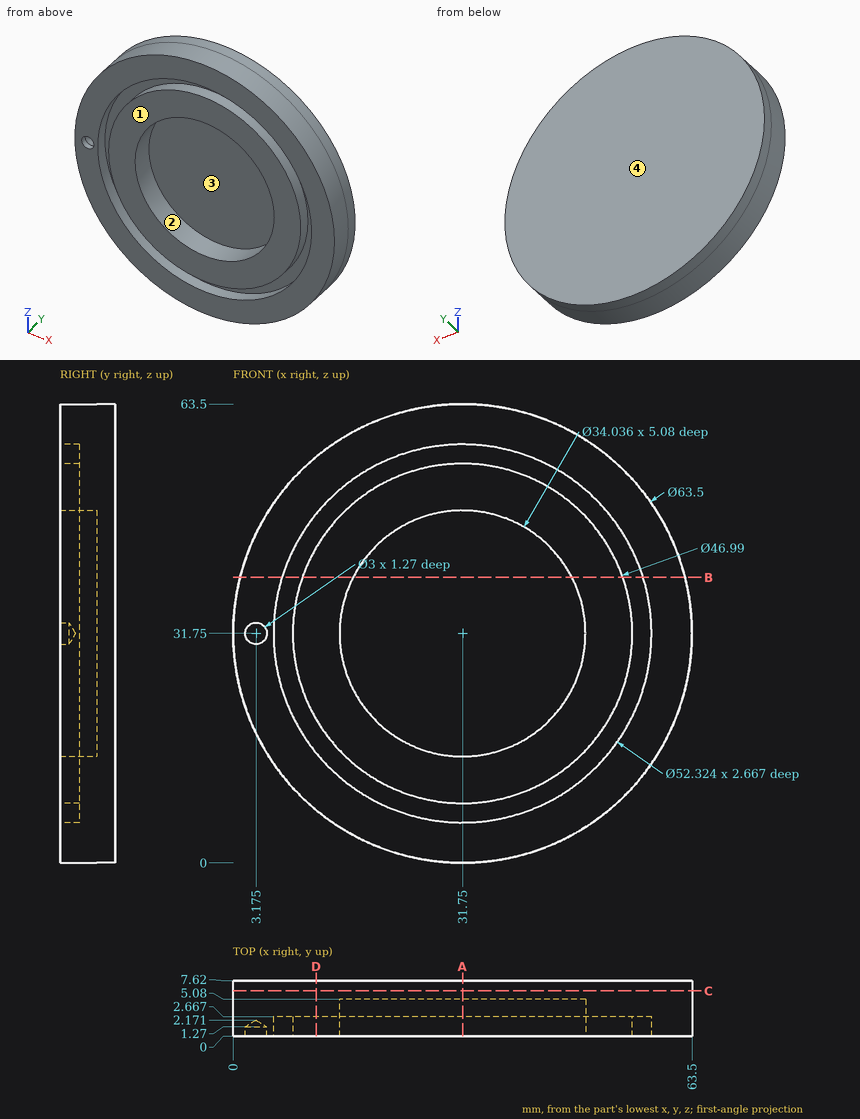
Geometry: see drawing. Coordinates: mm, zero at the bounding-box minimum. A direction names the side the tool comes from. Coordinates: 2 decimals unless noted, no trailing zeros. Order: outer loops, then holes, each group sorted by start corner. A loop starts at its lowest first (then second) coordinate and runs counter-clockwise, first axis right, second up. Notation, with made-up numbers: M 65.25,-15 L 83.25,-15 A30 cw 83.25,14 Z; hole C 72.25,-19.5 d6. An arc over 180 degrees is marked long. Answer as CSV lines item,"result".
1. Material intervals for line 1 (Z direction, x = 31.75, y = 3.3); line 2 (Z direction, x = 52, y = 2) (1 decimal); line 3 (Y direction, x = 23, z = 33.5), sorted ascending. Write a range as from..to.
Reported:
line 1,"0..14.73, 48.77..63.5"
line 2,"7.3..15.2, 19.8..43.7, 48.3..56.2"
line 3,"5.08..7.62"
2. Section A-A (x = 31.75). Return the cut outline in (y, z) (1 decimal), then the cut area to 3 significant figures.
Reported:
outline,"M 0,0 L 7.6,0 L 7.6,63.5 L 0,63.5 L 0,57.9 L 2.7,57.9 L 2.7,55.2 L 0,55.2 L 0,48.8 L 5.1,48.8 L 5.1,14.7 L 0,14.7 L 0,8.3 L 2.7,8.3 L 2.7,5.6 L 0,5.6 Z"
area,"297 mm2"
3. Access query for the marked faces 1 and 2. Directions: +Z, -Z, +X, -X, +Y, -Y. A direction counts if a zero-diameter tool reaches every point of the face in a straight line with its end or side. Return the directions, or none.
Reported:
face 1,"+Z, -Z, +X, -X, -Y"
face 2,"-Y"
4. Section D-D (x = 11.5). Return the cut outline in (y, z) (1 decimal), then the cut area to 3 significant figures.
Reported:
outline,"M 0,7.3 L 7.6,7.3 L 7.6,56.2 L 0,56.2 L 0,48.3 L 2.7,48.3 L 2.7,43.7 L 0,43.7 L 0,19.8 L 2.7,19.8 L 2.7,15.2 L 0,15.2 Z"
area,"348 mm2"
5. Section B-B (z = 39.5). Return the cut outline in (x, y), then the cut area to 3 significant figures.
Reported:
outline,"M 0.96,0 L 6.76,0 L 6.76,2.67 L 9.57,2.67 L 9.57,0 L 16.6,0 L 16.6,5.08 L 46.9,5.08 L 46.9,0 L 53.93,0 L 53.93,2.67 L 56.74,2.67 L 56.74,0 L 62.54,0 L 62.54,7.62 L 0.96,7.62 Z"
area,"300 mm2"
6. First-contact query: P1, Ø2, axis at x = 24, z = 31.5, coming from the -Y side; P2, Ø15.5, axis at x = 30, z = 42.5, coming from the -Y side; P3, Ø1.5, axis at x = 43.5, y = 5.5, coming from the -Z side; P4, Ø1, axis at y = 1.5, z = 34, coming from the -X side. Flat tips, straight axial feed; report the tip coordinate or a pass-through.
Reported:
P1,"y = 5.08"
P2,"y = 0"
P3,"z = 1.97"
P4,"x = 0.05"
7. Section C-C (y = 6.25). Return the cut outline in (x, z), then the cut area to 3 significant figures.
Reported:
outline,"C 31.75,31.75 d63.5"
area,"3,170 mm2"
8. Pull-direction query (Z, two-part tool) for the marked faces 3 and 4; classes: released by +Z, released by -Z, zero draft, split by the parting line, or undercut.
Reported:
face 3,"undercut"
face 4,"zero draft"
